Part print with two shaded views. Sizes in mm from the minimum x, y, z corner. A direction names the side the tool comes from. Round coordinates to 2 decimals unless told otherwise and drop trailing zeros. Order: outer loops, then holes, each group sorted by start corner. A loop starts at its lowest first (then second) coordinate and runs counter-clockwise, first axis right, second up. Notation, with made-up numbers: (74.25, 27.25) -> (85.25, 27.25) arc R18 cw to (85.25, 53.25) -> close; hole circle Ø10 at (-27.5, 64). An arc over 180 degrees is marked (long way). Answer as a JSON object with one key per item and string values.
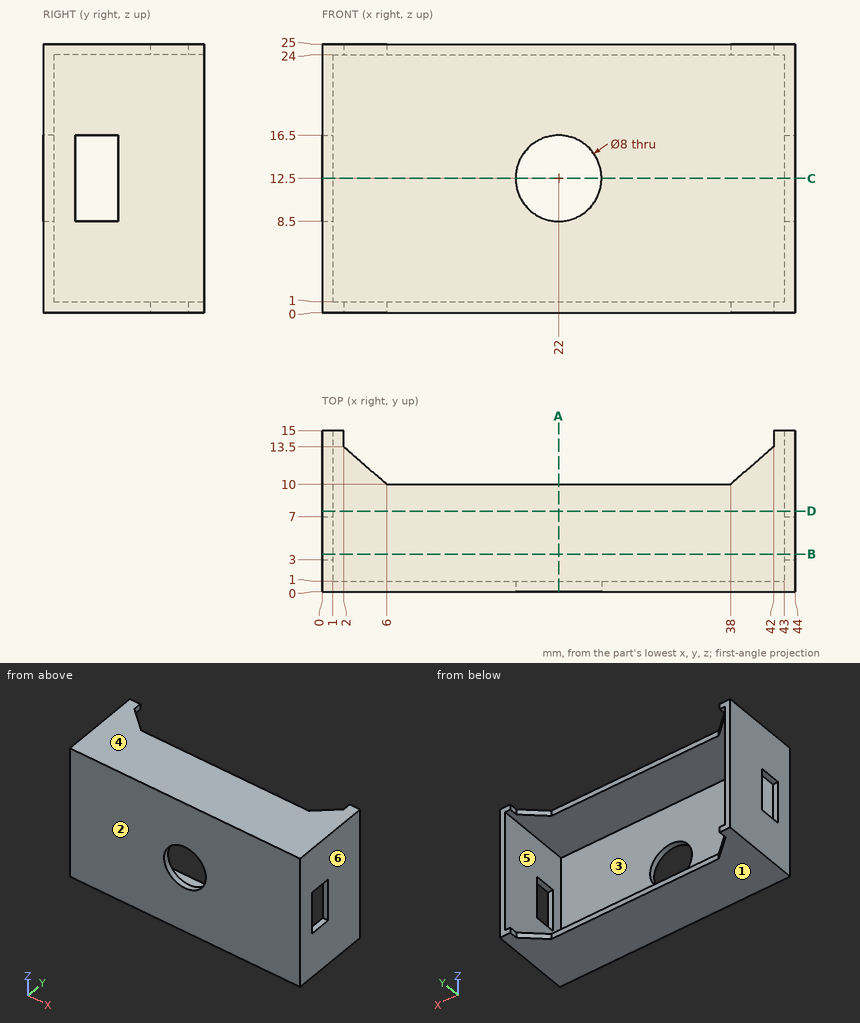
1) Cut at D-D, the plane y = 7.5. Give the cut face in (x, z).
Checked values:
{"outline": "(0, 0) -> (44, 0) -> (44, 25) -> (0, 25) -> close; hole (1, 1) -> (43, 1) -> (43, 24) -> (1, 24) -> close"}
2) Which spindle directions (+Z, -Z, +X, -X, +Y, -Y) get a long thin tool onto all of the face, cutting with end or side? Do the marked faces 5 and 6. Say none if no direction does.
Checked values:
{"face 5": "+Y", "face 6": "+Z, -Z, +X, +Y, -Y"}
3) Probe L1, parallel to Z at x = 33.5, y = 4.75; L2, parallel to X at y = 0.75, z = 12.5; L3, parallel to X at y = 8, z = 6.5. List the from-to ranges inside material, lowest first. Write a range as from..to.
Checked values:
{"L1": "z = 0..1, 24..25", "L2": "x = 0..18, 26..44", "L3": "x = 0..1, 43..44"}
4) Cut at C-C, the plane z = 12.5. Give the cut face in (x, y).
Checked values:
{"outline": "(0, 0) -> (18, 0) -> (18, 1) -> (1, 1) -> (1, 3) -> (0, 3) -> close; (0, 7) -> (1, 7) -> (1, 15) -> (0, 15) -> close; (26, 0) -> (44, 0) -> (44, 3) -> (43, 3) -> (43, 1) -> (26, 1) -> close; (43, 7) -> (44, 7) -> (44, 15) -> (43, 15) -> close"}
5) Cut at B-B, the plane y = 3.5. Give the cut face in (x, z).
Checked values:
{"outline": "(0, 0) -> (44, 0) -> (44, 8.5) -> (43, 8.5) -> (43, 1) -> (1, 1) -> (1, 8.5) -> (0, 8.5) -> close; (0, 16.5) -> (1, 16.5) -> (1, 24) -> (43, 24) -> (43, 16.5) -> (44, 16.5) -> (44, 25) -> (0, 25) -> close"}
6) Pull direction Z, two halves, no side cores. Call the marked faces 1, 2, 3 and 4: pulls with the +Z half, pulls with the -Z half, needs draft (parallel to the pull), parting line crosses it, or undercut.
Checked values:
{"face 1": "pulls with the -Z half", "face 2": "needs draft", "face 3": "undercut", "face 4": "pulls with the +Z half"}
7) Flat gauge pin, fed straight in: pin 1 Ø2 at (x, z) = (26.5, 9) entering from +Y. Where does the tip first touch, or does it go through?
Checked values:
{"pin 1": "stops at y = 1"}
8) Cut at A-A, the plane x = 22. Give the cut face in (y, z).
Checked values:
{"outline": "(0, 0) -> (10, 0) -> (10, 1) -> (1, 1) -> (1, 8.5) -> (0, 8.5) -> close; (0, 16.5) -> (1, 16.5) -> (1, 24) -> (10, 24) -> (10, 25) -> (0, 25) -> close"}
